Design review of the part built by this model. Coordinates are the model's own, in mm. A direction names the side the tool comes from. Coordinates: 2 decimals unless noted, no trailing zeros. Loops run counter-clockwise (first coordinate to the right, second up) from the corner with the lowest first, then second, coordinate; pieces in that order, holes last. Notation, with made-up numbers: (37, 25.5) - (93, 25.5) arc R16 cw to (93, 43.5) - close; hole circle Ø7 at (8, -5). An arc over 180 degrees is marked (long way). Return JSON: item names as keys, results as strings. Group by question number.
from build123d import *

# Parameters (mm, degrees)
CROQUIS1_W              = 350
CROQUIS1_H              = 63.65
SALIENTE_EXTRUIR1_DEPTH = 6.35
CROQUIS2_W              = 6.35
CROQUIS2_H              = 20
SALIENTE_EXTRUIR2_DEPTH = 6.35
CROQUIS3_W              = 20
CROQUIS3_H              = 6.35
SALIENTE_EXTRUIR3_DEPTH = 6.35


with BuildPart() as part:
    # Croquis1 → Saliente-Extruir1 (new body)
    with BuildSketch(Plane(origin=(0, 0, 0), x_dir=(-1, 0, 0), z_dir=(0, 0, 1))):
        with Locations((-18.650000026, -38.175)):
            Rectangle(CROQUIS1_W, CROQUIS1_H)
    extrude(amount=SALIENTE_EXTRUIR1_DEPTH)

    # Croquis2 → Saliente-Extruir2 (add)
    with BuildSketch(Plane.ZY.offset(156.349999974)):
        with Locations((3.175, 38.175)):
            Rectangle(CROQUIS2_W, CROQUIS2_H)
    saliente_extruir2 = extrude(amount=SALIENTE_EXTRUIR2_DEPTH)

    # Simetría1: Saliente-Extruir2 across plane
    add(saliente_extruir2.mirror(Plane(origin=(18.650000026, 0, 0), x_dir=(0, 0, 1), z_dir=(1, 0, 0))))

    # Croquis3 → Saliente-Extruir3 (add)
    with BuildSketch(Plane(origin=(0, 70, 0), x_dir=(1, 0, 0), z_dir=(0, 1, 0))):
        with Locations((18.650000026, -3.175)):
            Rectangle(CROQUIS3_W, CROQUIS3_H)
        with Locations((108.650000026, -3.175)):
            Rectangle(CROQUIS3_W, CROQUIS3_H)
        with Locations((-71.349999974, -3.175)):
            Rectangle(CROQUIS3_W, CROQUIS3_H)
    saliente_extruir3 = extrude(amount=SALIENTE_EXTRUIR3_DEPTH)

    # Simetría2: Saliente-Extruir3 across plane
    add(saliente_extruir3.mirror(Plane.ZX.offset(38.175)))


solid = part.part
Item 1: Draft analysis for pull direction X (two halves, no side actions). For faces 5 (the face through (28.65, 3, 3)), 6 (the face through (118.65, 3, 3)), 7 (the face through (8.65, 3, 3)), 8 (the face through (19, 76.35, 3)), state which applies: pulls with the +X half, pulls with the -X half, needs draft (parallel to the pull), parting line crosses it, or undercut.
Item 2: For P1, Ø3, axis at x = -158, z = 2, coming from the +Y side (3 decimals); P2, Ø1, axis at y = 18.5, z = 3, coming from the +X side; P3, Ø3, axis at y = 2, z = 2, coming from the +X side, all flat-tipped, find the tip position at first contact; note any pin that passes through.
Item 3: Add section B-B (y = 60). State the section outline as (x, z) points.
Item 4: Add section A-A (x = 40.5). State the section outline as (y, z) points.
Item 5: For faces 1 (the face through (-26, 6.35, 3)), 2 (the face through (8.65, 73, 3)), 3 (the face through (193.65, 59, 3)), 4 (the face through (-156.35, 17, 3)), list the 3-axis set-ups (+Z, -Z, +X, -X, +Y, -Y) from which the entire face can be reached by the end or side of a thin tool; tool diameter is ignored.
Item 6: To check wall thickness, follow line 1 (Y direction, x = 122, z = 6.25); line 2 (X direction, y = 64, z = 2.5). State the ranges of each line that lie inside material, in increasing order. Write a range as from..to.
Answers below:
{
 "1": {"face 5": "undercut", "face 6": "pulls with the +X half", "face 7": "undercut", "face 8": "needs draft"},
 "2": {"P1": "stops at y = 48.175", "P2": "stops at x = 193.65", "P3": "stops at x = 118.65"},
 "3": {"outline": "(-156.35, 0) - (193.65, 0) - (193.65, 6.35) - (-156.35, 6.35) - close"},
 "4": {"outline": "(6.35, 0) - (70, 0) - (70, 6.35) - (6.35, 6.35) - close"},
 "5": {"face 1": "+Z, -Z, -Y", "face 2": "+Z, -Z, +Y", "face 3": "+Z, -Z, +X, +Y", "face 4": "+Z, -Z, -X, -Y"},
 "6": {"line 1": "y = 6.35..70", "line 2": "x = -156.35..193.65"}
}
